```python
from build123d import *

# Parameters (mm, degrees)
POCKET_DEPTH      = 102.450988
POCKET_DEPTH_BACK = 126.450988
HOLE_D            = 3.4
HOLE_CBORE_D      = 6
HOLE_CBORE_DEPTH  = 3.1


with BuildPart() as part:
    # Sketch → Revolution (revolve)
    with BuildSketch(Plane.XZ):
        Polygon((16, 0), (16, 5), (7.5, 5), (7.5, 24), (4, 24), (4, 0), align=None)
    revolve(axis=Axis((0, 0, 0), (0, 0, 1)))

    # Sketch001 → Pocket (cut, two sides)
    with BuildSketch(Plane.XY) as pocket_sk:
        Polygon((10.5, 20), (50.5, 20), (50.5, -20), (10.5, -20), (10.5, 0), align=None)
    pocket = extrude(amount=-POCKET_DEPTH, mode=Mode.SUBTRACT) + extrude(pocket_sk.sketch, amount=POCKET_DEPTH_BACK, mode=Mode.SUBTRACT)

    # Mirrored: Pocket across Sketch001 V_Axis
    add(pocket.mirror(Plane(origin=(0, 0, 0), x_dir=(0, 0, 1), z_dir=(1, 0, 0))), mode=Mode.SUBTRACT)

    # Hole (through all)
    with Locations(Plane(origin=(0, 0, 0), x_dir=(1, 0, 0), z_dir=(0, 0, -1))):
        with Locations((0, -12), (0, 12)):
            CounterBoreHole(HOLE_D / 2, HOLE_CBORE_D / 2, HOLE_CBORE_DEPTH)


solid = part.part
```
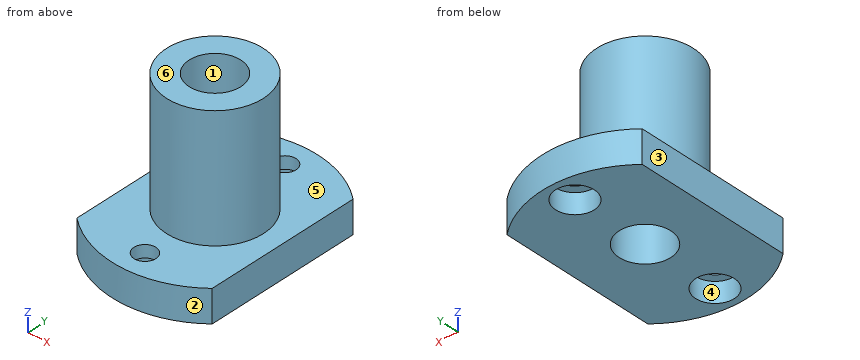
CAD build for the part. Positions are in the model's coordinates, mm. Face numbers are marked on the shaded views. A direction names the side the tool comes from. Round coordinates to 2 decimals unless told otherwise and drop trailing zeros. Order: outer loops, then holes, each group sorted by start corner. A loop starts at its lowest first (then second) coordinate and runs counter-clockwise, first axis right, second up.
Item 1: Saw through at B-B on z = 2. Write the cut outline in (x, y).
Item 2: Saw through at D-D on x = 3.5. Write the cut outline in (y, z).
Item 3: Mould opens along Y. For the marked faces 1, 2 and 3 say: pulls with the +Y half, pulls with the -Y half, needs draft (parallel to the pull), parting line crosses it, or undercut.
Item 4: Saw through at C-C on y = 0. Write the cut outline in (x, z), then the cut area to 3 significant figures.
Item 5: Saw through at A-A on x = 0. Write the cut outline in (y, z), then the cut area to 3 significant figures.
Item 6: Tool access for the marked faces 4, 5 and 6: list every direction of +Z, -Z, +X, -X, +Y, -Y with a clear straight run to the whole face (end or side of a thin tool).
Item 7: Pin check, flat tips, straight feed: pin 1 (8 mm diameter, centred on x = 0, y = -12, fed in from +Z); pin 2 (8 mm diameter, centred on x = 4.5, z = 21, fed in from -Y); pin 3 (1.5 mm diameter, centred on y = 9, z = 17, fed in from +X); pin 4 (12 mm diameter, centred on x = -7.5, z = 14.5, fed in from -Y). Stop position of each tip, or through.
Item 8: Probe line 1 along Y through (x, z) = (0, 14.25); line 2 along X through (y, z) = (-12, 1.25); line 3 along X through (y, z) = (12, 3.8). List the from-to ranges inside material, lowest first.
Reported:
1. outline: (-10.5, -12.07) arc R16 ccw to (10.5, -12.07) - (10.5, 12.07) arc R16 ccw to (-10.5, 12.07) - close; hole circle Ø8 at (0, 0); hole circle Ø6 at (0, -12); hole circle Ø6 at (0, 12)
2. outline: (-15.61, 0) - (-1.94, 0) - (-1.94, 24) - (-6.63, 24) - (-6.63, 5) - (-15.61, 5) - close; (1.94, 0) - (15.61, 0) - (15.61, 5) - (6.63, 5) - (6.63, 24) - (1.94, 24) - close
3. face 1: undercut
3. face 2: pulls with the -Y half
3. face 3: needs draft
4. outline: (-10.5, 0) - (-4, 0) - (-4, 24) - (-7.5, 24) - (-7.5, 5) - (-10.5, 5) - close; (4, 0) - (10.5, 0) - (10.5, 5) - (7.5, 5) - (7.5, 24) - (4, 24) - close
4. area: 198 mm2
5. outline: (-16, 0) - (-15, 0) - (-15, 3.1) - (-13.7, 3.1) - (-13.7, 5) - (-16, 5) - close; (-10.3, 3.1) - (-9, 3.1) - (-9, 0) - (-4, 0) - (-4, 24) - (-7.5, 24) - (-7.5, 5) - (-10.3, 5) - close; (4, 0) - (9, 0) - (9, 3.1) - (10.3, 3.1) - (10.3, 5) - (7.5, 5) - (7.5, 24) - (4, 24) - close; (13.7, 3.1) - (15, 3.1) - (15, 0) - (16, 0) - (16, 5) - (13.7, 5) - close
5. area: 203 mm2
6. face 4: -Z
6. face 5: +Z
6. face 6: +Z, +X, -X, +Y, -Y
7. pin 1: stops at z = 5
7. pin 2: stops at y = -7.48
7. pin 3: passes through
7. pin 4: stops at y = -7.35
8. line 1: y = -7.5 to -4, 4 to 7.5
8. line 2: x = -10.5 to -3, 3 to 10.5
8. line 3: x = -10.5 to -1.7, 1.7 to 10.5
